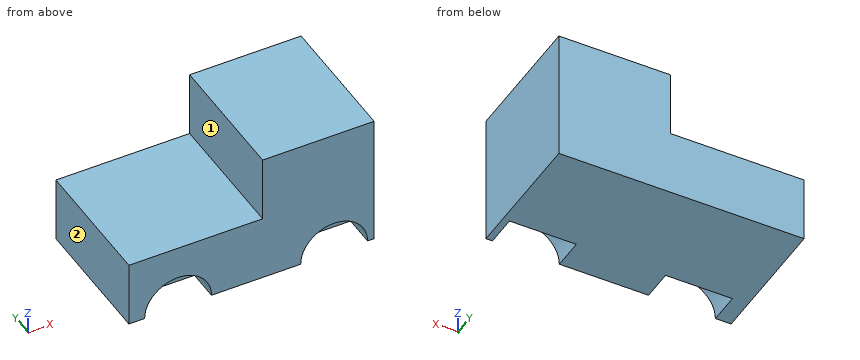
from build123d import *

# Parameters (mm, degrees)
F0_W     = 55
F0_H     = 30
F1_DEPTH = 30
F2_W     = 30
F2_H     = 15
F3_DEPTH = 30.001
F5_DEPTH = 7


with BuildPart() as f1:
    # F0 (on Front) → F1 (new body)
    with BuildSketch(Plane.XZ):
        with Locations((-31.4610829165, -24.9669793993)):
            Rectangle(F0_W, F0_H)
    extrude(amount=F1_DEPTH)

    # F2 (on face) → F3 (cut, through all)
    with BuildSketch(Plane.XZ.offset(30)):
        with Locations((-43.9610829165, -17.4669793993)):
            Rectangle(F2_W, F2_H)
    extrude(amount=-F3_DEPTH, mode=Mode.SUBTRACT)

    # F4 (on face) → F5 (cut)
    with BuildSketch(Plane.XZ.offset(30)):
        with BuildLine():
            Line((-55.4294285178, -39.9669793993), (-40.4294285178, -39.9669793993))
            ThreePointArc((-40.4294285178, -39.9669793993), (-47.9294285178, -32.4669793993), (-55.4294285178, -39.9669793993))
        make_face()
        with BuildLine():
            ThreePointArc((-5.4294285178, -39.9669793993), (-12.9294285178, -32.4669793993), (-20.4294285178, -39.9669793993))
            Line((-20.4294285178, -39.9669793993), (-5.4294285178, -39.9669793993))
        make_face()
    extrude(amount=-F5_DEPTH, mode=Mode.SUBTRACT)


solid = f1.part
CAD build for the part. Positions are in the model's coordinates, mm. Face numbers are marked on the shaded views. A direction names the side the tool comes from. Coordinates: 2 decimals unless noted, no trailing zeros. Loops run counter-clockwise (first coordinate to the right, second up) from the corner with the lowest first, then second, coordinate; pieces in that order, holes last. Notation, with made-up numbers: (82, 29.25) - (95, 29.25) arc R27 ccw to (95, 50.25) - close; hole circle Ø3 at (-17, 21). An arc over 180 degrees is marked (long way). Use one line per item in the form item = value. Start each with the question number.
1) Band-saw the part on B-B (z = -19.75). Give the cut face in (x, y), and give its area (3 significant figures).
2) Band-saw the part on D-D (y = -15.5). Give the cut face in (x, z), and give its area (3 significant figures).
3) Drill centre lines: L1, parallel to Z at x = -41.5, y = -1.25; L2, parallel to X at y = -23.25, z = -15; L3, parallel to X at y = -28.5, z = -37. Where is each one in solid material? Low to high. Write a range as from..to.
4) Band-saw the part on A-A (y = -25.25). Give the cut face in (x, z), and give its area (3 significant figures).
5) Band-saw the part on C-C (x = -10). Give the cut face in (y, z).
6) Tool access for the marked faces 1 and 2: list every direction of +Z, -Z, +X, -X, +Y, -Y with a clear straight run to the whole face (end or side of a thin tool).
7) Flat gauge pins, fed straight in: pin 1 (4.5 mm diameter, centred on y = -16, z = -20, fed in from -X); pin 2 (10 mm diameter, centred on x = -38, y = -5.5, fed in from +Z); pin 3 (2 mm diameter, centred on x = -46, z = -35, fed in from -Y). Where does each tip first touch, or does it go through?
Check values:
q1.outline = (-28.96, -30) - (-3.96, -30) - (-3.96, 0) - (-28.96, 0) - close
q1.area = 750 mm2
q2.outline = (-58.96, -39.97) - (-3.96, -39.97) - (-3.96, -9.97) - (-28.96, -9.97) - (-28.96, -24.97) - (-58.96, -24.97) - close
q2.area = 1,200 mm2
q3.L1 = -39.97..-24.97
q3.L2 = -28.96..-3.96
q3.L3 = -58.96..-54.82, -41.04..-19.82, -6.04..-3.96
q4.outline = (-58.96, -39.97) - (-55.43, -39.97) arc R7.5 cw to (-40.43, -39.97) - (-20.43, -39.97) arc R7.5 cw to (-5.43, -39.97) - (-3.96, -39.97) - (-3.96, -9.97) - (-28.96, -9.97) - (-28.96, -24.97) - (-58.96, -24.97) - close
q4.area = 1,020 mm2
q5.outline = (-30, -33.06) - (-23, -33.06) - (-23, -39.97) - (0, -39.97) - (0, -9.97) - (-30, -9.97) - close
q6.face_1 = +Z, -X, +Y, -Y
q6.face_2 = +Z, -Z, -X, +Y, -Y
q7.pin_1 = -28.96
q7.pin_2 = -24.97
q7.pin_3 = -23
